Work out the finished part from the listing and answer in its coordinate system (mm). A direction names the side the tool comes from. Coordinates: 2 decimals unless noted, no trailing zeros. Write each loop counter-clockwise with the first axis right and the second up, starting at its lowest first coordinate (ties: lowest second). Pieces come first, ordered by that corner, then holes. Notation, with made-up numbers: (63, 28.25) - (72, 28.25) arc R29 cw to (72, 50.25) - close; hole circle Ø4 at (-37.5, 1). An arc over 180 degrees is marked (long way). One line per item, written item: value.
```python
from build123d import *

# Parameters (mm, degrees)
SKETCH1_R                                      = 38.1
BOSS_EXTRUDE1_DEPTH                            = 6.35
CBORE_FOR_4_BUTTON_HEAD_CAP_SCREW1_D           = 2.8702
CBORE_FOR_4_BUTTON_HEAD_CAP_SCREW1_CBORE_D     = 4.826
CBORE_FOR_4_BUTTON_HEAD_CAP_SCREW1_CBORE_DEPTH = 1.905
CIRPATTERN1_COUNT                              = 8
SKETCH7_R                                      = 0.3937
SKETCH7_R_2                                    = 0.5969
SKETCH7_R_3                                    = 0.8001
SKETCH7_R_4                                    = 0.79375
CUT_EXTRUDE1_DEPTH                             = 7.35
CIRPATTERN3_COUNT                              = 12
CUT_EXTRUDE3_REACH                             = 8.35
SKETCH8_R                                      = 0.396875
CUT_EXTRUDE4_REACH                             = 8.35
SKETCH9_R                                      = 0.396875


with BuildPart() as part:
    # Sketch1 → Boss-Extrude1 (new body)
    with BuildSketch(Plane(origin=(0, 0, 0), x_dir=(1, 0, 0), z_dir=(0, 1, 0))):
        Circle(SKETCH1_R)
    extrude(amount=BOSS_EXTRUDE1_DEPTH)

    # CBORE for #4 Button Head Cap Screw1 (through all)
    with Locations(Plane(origin=(0, 0, 0), x_dir=(-1, 0, 0), z_dir=(0, -1, 0))):
        with Locations((0, -33.3375)):
            cbore_for_4_button_head_cap_screw1 = CounterBoreHole(CBORE_FOR_4_BUTTON_HEAD_CAP_SCREW1_D / 2, CBORE_FOR_4_BUTTON_HEAD_CAP_SCREW1_CBORE_D / 2, CBORE_FOR_4_BUTTON_HEAD_CAP_SCREW1_CBORE_DEPTH)

    # CirPattern1: CBORE for #4 Button Head Cap Screw1 ×8 about axis
    cirpattern1_axis = Axis((0, 0, 0), (0, 1, 0))
    for i in range(1, CIRPATTERN1_COUNT):
        add(cbore_for_4_button_head_cap_screw1.rotate(cirpattern1_axis, i * 360 / CIRPATTERN1_COUNT), mode=Mode.SUBTRACT)

    # Sketch7 → Cut-Extrude1 (cut, through all)
    with BuildSketch(Plane.XZ):
        with Locations((0, 12.7)):
            Circle(SKETCH7_R)
        with Locations((0, 9.525)):
            Circle(SKETCH7_R_2)
        with Locations((0, 5.715)):
            Circle(SKETCH7_R_3)
        Circle(SKETCH7_R_4)
    cut_extrude1 = extrude(amount=-CUT_EXTRUDE1_DEPTH, mode=Mode.SUBTRACT)

    # CirPattern3: Cut-Extrude1 ×12 about axis
    cirpattern3_axis = Axis((0, 0, 0), (0, 1, 0))
    for i in range(1, CIRPATTERN3_COUNT):
        add(cut_extrude1.rotate(cirpattern3_axis, i * 360 / CIRPATTERN3_COUNT), mode=Mode.SUBTRACT)

    # Sketch8 → Cut-Extrude3 (cut, up to next)
    with BuildSketch(Plane(origin=(0, 6.35, 0), x_dir=(1, 0, 0), z_dir=(0, 1, 0)), mode=Mode.PRIVATE) as cut_extrude3_sk1:
        with Locations((3.368817958, 0)):
            Circle(SKETCH8_R)
    cut_extrude3_tool1 = extrude(cut_extrude3_sk1.sketch, amount=-CUT_EXTRUDE3_REACH, mode=Mode.PRIVATE) & part.part
    add(cut_extrude3_tool1.solids().sort_by_distance((3.368818, 6.35, 0))[0], mode=Mode.SUBTRACT)
    # Sketch8 → Cut-Extrude3 (cut, up to next)
    with BuildSketch(Plane(origin=(0, 6.35, 0), x_dir=(1, 0, 0), z_dir=(0, 1, 0)), mode=Mode.PRIVATE) as cut_extrude3_sk2:
        with Locations((2.382114023, -2.382114023)):
            Circle(SKETCH8_R)
    cut_extrude3_tool2 = extrude(cut_extrude3_sk2.sketch, amount=-CUT_EXTRUDE3_REACH, mode=Mode.PRIVATE) & part.part
    add(cut_extrude3_tool2.solids().sort_by_distance((2.382114, 6.35, 2.382114))[0], mode=Mode.SUBTRACT)
    # Sketch8 → Cut-Extrude3 (cut, up to next)
    with BuildSketch(Plane(origin=(0, 6.35, 0), x_dir=(1, 0, 0), z_dir=(0, 1, 0)), mode=Mode.PRIVATE) as cut_extrude3_sk3:
        with Locations((0, -3.368817958)):
            Circle(SKETCH8_R)
    cut_extrude3_tool3 = extrude(cut_extrude3_sk3.sketch, amount=-CUT_EXTRUDE3_REACH, mode=Mode.PRIVATE) & part.part
    add(cut_extrude3_tool3.solids().sort_by_distance((0, 6.35, 3.368818))[0], mode=Mode.SUBTRACT)
    # Sketch8 → Cut-Extrude3 (cut, up to next)
    with BuildSketch(Plane(origin=(0, 6.35, 0), x_dir=(1, 0, 0), z_dir=(0, 1, 0)), mode=Mode.PRIVATE) as cut_extrude3_sk4:
        with Locations((-2.382114023, -2.382114023)):
            Circle(SKETCH8_R)
    cut_extrude3_tool4 = extrude(cut_extrude3_sk4.sketch, amount=-CUT_EXTRUDE3_REACH, mode=Mode.PRIVATE) & part.part
    add(cut_extrude3_tool4.solids().sort_by_distance((-2.382114, 6.35, 2.382114))[0], mode=Mode.SUBTRACT)
    # Sketch8 → Cut-Extrude3 (cut, up to next)
    with BuildSketch(Plane(origin=(0, 6.35, 0), x_dir=(1, 0, 0), z_dir=(0, 1, 0)), mode=Mode.PRIVATE) as cut_extrude3_sk5:
        with Locations((-3.368817958, 0)):
            Circle(SKETCH8_R)
    cut_extrude3_tool5 = extrude(cut_extrude3_sk5.sketch, amount=-CUT_EXTRUDE3_REACH, mode=Mode.PRIVATE) & part.part
    add(cut_extrude3_tool5.solids().sort_by_distance((-3.368818, 6.35, 0))[0], mode=Mode.SUBTRACT)
    # Sketch8 → Cut-Extrude3 (cut, up to next)
    with BuildSketch(Plane(origin=(0, 6.35, 0), x_dir=(1, 0, 0), z_dir=(0, 1, 0)), mode=Mode.PRIVATE) as cut_extrude3_sk6:
        with Locations((-2.382114023, 2.382114023)):
            Circle(SKETCH8_R)
    cut_extrude3_tool6 = extrude(cut_extrude3_sk6.sketch, amount=-CUT_EXTRUDE3_REACH, mode=Mode.PRIVATE) & part.part
    add(cut_extrude3_tool6.solids().sort_by_distance((-2.382114, 6.35, -2.382114))[0], mode=Mode.SUBTRACT)
    # Sketch8 → Cut-Extrude3 (cut, up to next)
    with BuildSketch(Plane(origin=(0, 6.35, 0), x_dir=(1, 0, 0), z_dir=(0, 1, 0)), mode=Mode.PRIVATE) as cut_extrude3_sk7:
        with Locations((0, 3.368817958)):
            Circle(SKETCH8_R)
    cut_extrude3_tool7 = extrude(cut_extrude3_sk7.sketch, amount=-CUT_EXTRUDE3_REACH, mode=Mode.PRIVATE) & part.part
    add(cut_extrude3_tool7.solids().sort_by_distance((0, 6.35, -3.368818))[0], mode=Mode.SUBTRACT)
    # Sketch8 → Cut-Extrude3 (cut, up to next)
    with BuildSketch(Plane(origin=(0, 6.35, 0), x_dir=(1, 0, 0), z_dir=(0, 1, 0)), mode=Mode.PRIVATE) as cut_extrude3_sk8:
        with Locations((2.382114023, 2.382114023)):
            Circle(SKETCH8_R)
    cut_extrude3_tool8 = extrude(cut_extrude3_sk8.sketch, amount=-CUT_EXTRUDE3_REACH, mode=Mode.PRIVATE) & part.part
    add(cut_extrude3_tool8.solids().sort_by_distance((2.382114, 6.35, -2.382114))[0], mode=Mode.SUBTRACT)

    # Sketch9 → Cut-Extrude4 (cut, up to next)
    with BuildSketch(Plane(origin=(0, 6.35, 0), x_dir=(1, 0, 0), z_dir=(0, 1, 0)), mode=Mode.PRIVATE) as cut_extrude4_sk1:
        with Locations((1.187739958, 1.187739958)):
            Circle(SKETCH9_R)
    cut_extrude4_tool1 = extrude(cut_extrude4_sk1.sketch, amount=-CUT_EXTRUDE4_REACH, mode=Mode.PRIVATE) & part.part
    add(cut_extrude4_tool1.solids().sort_by_distance((1.18774, 6.35, -1.18774))[0], mode=Mode.SUBTRACT)
    # Sketch9 → Cut-Extrude4 (cut, up to next)
    with BuildSketch(Plane(origin=(0, 6.35, 0), x_dir=(1, 0, 0), z_dir=(0, 1, 0)), mode=Mode.PRIVATE) as cut_extrude4_sk2:
        with Locations((1.622482956, -0.434742998)):
            Circle(SKETCH9_R)
    cut_extrude4_tool2 = extrude(cut_extrude4_sk2.sketch, amount=-CUT_EXTRUDE4_REACH, mode=Mode.PRIVATE) & part.part
    add(cut_extrude4_tool2.solids().sort_by_distance((1.622483, 6.35, 0.434743))[0], mode=Mode.SUBTRACT)
    # Sketch9 → Cut-Extrude4 (cut, up to next)
    with BuildSketch(Plane(origin=(0, 6.35, 0), x_dir=(1, 0, 0), z_dir=(0, 1, 0)), mode=Mode.PRIVATE) as cut_extrude4_sk3:
        with Locations((0.434742998, -1.622482956)):
            Circle(SKETCH9_R)
    cut_extrude4_tool3 = extrude(cut_extrude4_sk3.sketch, amount=-CUT_EXTRUDE4_REACH, mode=Mode.PRIVATE) & part.part
    add(cut_extrude4_tool3.solids().sort_by_distance((0.434743, 6.35, 1.622483))[0], mode=Mode.SUBTRACT)
    # Sketch9 → Cut-Extrude4 (cut, up to next)
    with BuildSketch(Plane(origin=(0, 6.35, 0), x_dir=(1, 0, 0), z_dir=(0, 1, 0)), mode=Mode.PRIVATE) as cut_extrude4_sk4:
        with Locations((-1.187739958, -1.187739958)):
            Circle(SKETCH9_R)
    cut_extrude4_tool4 = extrude(cut_extrude4_sk4.sketch, amount=-CUT_EXTRUDE4_REACH, mode=Mode.PRIVATE) & part.part
    add(cut_extrude4_tool4.solids().sort_by_distance((-1.18774, 6.35, 1.18774))[0], mode=Mode.SUBTRACT)
    # Sketch9 → Cut-Extrude4 (cut, up to next)
    with BuildSketch(Plane(origin=(0, 6.35, 0), x_dir=(1, 0, 0), z_dir=(0, 1, 0)), mode=Mode.PRIVATE) as cut_extrude4_sk5:
        with Locations((-1.622482956, 0.434742998)):
            Circle(SKETCH9_R)
    cut_extrude4_tool5 = extrude(cut_extrude4_sk5.sketch, amount=-CUT_EXTRUDE4_REACH, mode=Mode.PRIVATE) & part.part
    add(cut_extrude4_tool5.solids().sort_by_distance((-1.622483, 6.35, -0.434743))[0], mode=Mode.SUBTRACT)
    # Sketch9 → Cut-Extrude4 (cut, up to next)
    with BuildSketch(Plane(origin=(0, 6.35, 0), x_dir=(1, 0, 0), z_dir=(0, 1, 0)), mode=Mode.PRIVATE) as cut_extrude4_sk6:
        with Locations((-0.434742998, 1.622482956)):
            Circle(SKETCH9_R)
    cut_extrude4_tool6 = extrude(cut_extrude4_sk6.sketch, amount=-CUT_EXTRUDE4_REACH, mode=Mode.PRIVATE) & part.part
    add(cut_extrude4_tool6.solids().sort_by_distance((-0.434743, 6.35, -1.622483))[0], mode=Mode.SUBTRACT)


solid = part.part
```
Item 1: Section C-C, the plane z = 20 is taken. Determine the outline of the cut face in (x, y), then the cut area to 3 significant figures.
Evaluation:
outline: (-32.43, 0) - (32.43, 0) - (32.43, 6.35) - (-32.43, 6.35) - close
area: 412 mm2
Item 2: Determine the mould class of faces 3 (the face through (-34.74, 4.16, -0.31)), 4 (the face through (8, 0, -1)), 5 (the face through (-30.235, 3.131, 23.183)), 6 (the face through (22, 1.905, 25)) for opening direction X: +X half, -X half, draft (parallel to the pull), parting line (faces both ways), or undercut.
Evaluation:
face 3: undercut
face 4: draft
face 5: parting line
face 6: undercut
Item 3: Given pin 1 (3.5 mm diameter, centred on x = 23.57, z = -23.57, fed in from +Y); pin 2 (1.1 mm diameter, centred on x = -8.25, z = -4.76, fed in from +Y); pin 3 (2 mm diameter, centred on x = 28.5, y = 1, fed in from -Z); pin 4 (1 mm diameter, centred on y = 1, z = 26, fed in from +X), each flat-ended and moving along its own axis, determine where each tip first touches the part or whether it passes through.
Evaluation:
pin 1: stops at y = 6.35
pin 2: passes through
pin 3: stops at z = -26.37
pin 4: stops at x = 28.31
Item 4: Section A-A, the plane y = 3 is taken. Give the number of separate pieces and of enclosed holes in the cut face, then the cut area to 3 significant figures.
Evaluation:
separate pieces: 1
enclosed holes: 59
area: 4,460 mm2
Item 5: Consider probe 1 along X at (y, z) = (2.25, 1.5); probe 2 along X at (y, z) = (0.75, 25); probe 3 along X at (y, z) = (4.75, -1). Determine where each line is inside the solid, lowest interval first.
Evaluation:
probe 1: x = -38.07 to -1.43, -0.94 to 0.06, 0.81 to 38.07
probe 2: x = -28.75 to -25.52, -21.63 to 21.63, 25.52 to 28.75
probe 3: x = -38.09 to -34.37, -32.31 to 0.84, 1.54 to 32.31, 34.37 to 38.09
Item 6: Which of the six approach directions +Z, -Z, +X, -X, +Y, -Y give full straight-line access (tool end or side, diameter ignored) to faces 1 (the face through (31.303, 0.939, 1.297)), 2 (the face through (-24.94, 4.16, -24.01))?
Evaluation:
face 1: -Y
face 2: +Y, -Y
Item 7: Section B-B, the plane x = -20 is taken. Determine the outline of the cut face in (y, z), then the cut area to 3 significant figures.
Evaluation:
outline: (0, -32.43) - (6.35, -32.43) - (6.35, 32.43) - (0, 32.43) - close
area: 412 mm2
